Work out the finished part from the listing and answer in its coordinate system (mm). A direction names the side the tool comes from. Coordinates: 2 decimals unless noted, no trailing zeros. Loops run counter-clockwise (first coordinate to the right, second up) from the corner with the lowest first, then second, coordinate; pieces in that order, holes last. Notation, with made-up numbers: M 7.5,-9 L 65.5,-9 A31 cw 65.5,19 Z; hole C -19,44 d9. An arc over 180 degrees is marked long. Write each question's results on one line, items separated by ' | '.
```python
from build123d import *

# Parameters (mm, degrees)
EXTRUDE2_DEPTH = 1.27
EXTRUDE3_DEPTH = 1.27
EXTRUDE4_DEPTH = 1.27


with BuildPart() as part:
    # Sketch2 → Extrude2 (new body)
    with BuildSketch(Plane.XY):
        with BuildLine():
            Line((25.4, 0), (167.299096948, 0))
            Line((167.299096948, 0), (167.299096948, 50.8))
            Line((167.299096948, 50.8), (25.4, 50.8))
            ThreePointArc((25.4, 50.8), (0, 25.4), (25.4, 0))
        make_face()
    extrude(amount=EXTRUDE2_DEPTH)

    # Sketch5 → Extrude3 (add)
    with BuildSketch(Plane.XY.offset(1.27)):
        with BuildLine():
            Line((25.4, 50.8), (37.759096935, 50.8))
            Line((37.759096935, 50.8), (36.934864936, 31.759918178))
            Line((36.934864936, 31.759918178), (25.187364936, 31.759918178))
            ThreePointArc((25.187364936, 31.759918178), (18.674313706, 25.683931539), (24.624718961, 19.055950907))
            Line((24.624718961, 19.055950907), (36.384918961, 19.055950907))
            Line((36.384918961, 19.055950907), (35.56, 0))
            Line((35.56, 0), (25.4, 0))
            ThreePointArc((25.4, 0), (0, 25.4), (25.4, 50.8))
        make_face()
    extrude(amount=EXTRUDE3_DEPTH)

    # Sketch5<4> → Extrude4 (add)
    with BuildSketch(Plane.XY.offset(1.27)):
        with BuildLine():
            Line((153.939033989, 35.56), (166.639033989, 35.56))
            Line((166.639033989, 35.56), (167.299096935, 50.8))
            Line((167.299096935, 50.8), (151.568912005, 50.8))
            ThreePointArc((151.568912005, 50.8), (144.541778303, 47.977914686), (141.418418385, 41.079407862))
            Line((141.418418385, 41.079407862), (141.206176472, 36.176536601))
            ThreePointArc((141.206176472, 36.176536601), (141.660521084, 32.217758839), (143.31923128, 28.594634375))
            Line((143.31923128, 28.594634375), (152.200348571, 15.24))
            Line((152.200348571, 15.24), (139.500348571, 15.24))
            Line((139.500348571, 15.24), (138.840285624, 0))
            Line((138.840285624, 0), (155.369404166, 0))
            ThreePointArc((155.369404166, 0), (162.396457641, 2.822008486), (165.519888176, 9.720370185))
            Line((165.519888176, 9.720370185), (165.683377481, 13.495126865))
            ThreePointArc((165.683377481, 13.495126865), (165.229082159, 17.454048315), (163.570334687, 21.077306532))
            Line((163.570334687, 21.077306532), (153.939033989, 35.56))
        make_face()
        Polygon((53.34, 50.8), (40.64, 50.8), (38.440216103, -0.015869084), (51.140216103, -0.015869084), (51.965822026, 19.055950907), (54.505822026, 19.055950907), (53.680316159, -0.013557756), (66.380816438, -0.002001116), (68.58, 50.8), (55.88, 50.8), (55.055768, 31.759918178), (52.515768, 31.759918178), align=None)
        Polygon((83.479096935, 50.8), (70.779096935, 50.8), (68.58, 0), (81.28, 0), align=None)
        Polygon((111.419096935, 50.8), (86.019096935, 50.8), (83.82, 0), (109.22, 0), (109.846156204, 14.464453409), (97.146156204, 14.464453409), (97.306540074, 18.16938358), (110.006540074, 18.16938358), (110.632696278, 32.633836988), (97.932696278, 32.633836988), (98.093080148, 36.33876716), (110.793080148, 36.33876716), align=None)
        Polygon((139.318340653, 50.8), (113.959096935, 50.8), (111.76, 0), (123.65404294, 0), (124.753591407, 25.4), (138.218792185, 25.4), (138.658714454, 35.562376595), (125.193513676, 35.562376595), (125.413217607, 40.637623405), (138.878418385, 40.637623405), align=None)
    extrude(amount=EXTRUDE4_DEPTH)


solid = part.part
```
1) Find section B-B, the plane z = 0.55. Give the vertices of the cut face in (x, y), and give its area (3 significant figures).
Check result:
outline: M 25.4,0 L 167.3,0 L 167.3,50.8 L 25.4,50.8 A25.4 ccw Z | area: 8,220 mm^2
2) Given pin 1 Ø1.7 at (x, y) = (52.5, 11) entering from +Z; pin 2 Ø1.3 at (x, z) = (78.5, 2) entering from -Y; pin 3 Ø0.6 at (x, z) = (53, 2) entering from -Y, each flat-ended and moving along its own axis, determine where each tip first touches the part or whether it passes through.
Check result:
pin 1: z = 1.27 | pin 2: y = 0 | pin 3: y = 19.06
3) Which of the six approach directions +Z, -Z, +X, -X, +Y, -Y give full straight-line access (tool end or side, diameter ignored) to faces 5 (the face through (162.32, 2.75, 1.9)), 6 (the face through (147.7, 22.01, 1.9)), 7 (the face through (144.62, 48.05, 1.9)), 8 (the face through (122, 31, 2.54)), 9 (the face through (164, 24, 1.27))?
Check result:
face 5: +Z, +X, -Y | face 6: +Z | face 7: +Z, +Y | face 8: +Z, +X, -X, +Y, -Y | face 9: +Z, +X
4) For a pull along X with two mould halves and no side action, classify faces 1 (the face through (158.82, 28.22, 1.9)), 2 (the face through (54, 41, 1.27)), 3 (the face through (15, 26, 2.54)), 4 (the face through (135, 20, 1.27)) as released by +X, released by -X, zero draft, split by the parting line, or undercut.
Check result:
face 1: released by +X | face 2: undercut | face 3: zero draft | face 4: undercut
5) Straight lines are drawn through the part: probe 1 along Y at (x, z) = (102, 2.25); probe 2 along X at (y, z) = (27, 2.2); probe 3 along Y at (x, z) = (142.5, 2.45). For each, find the intervals that lie inside material, in ascending order. Write a range as [from, to].
Check result:
probe 1: [0, 14.46], [18.17, 32.63], [36.34, 50.8] | probe 2: [0.05, 18.87], [39.61, 67.55], [69.75, 82.45], [84.99, 110.39], [112.93, 138.29], [144.38, 159.63] | probe 3: [0, 15.24], [30.02, 45.22]
6) Find section A-A, the plane x = 136.5. Give the vertices of the cut face in (y, z).
Check result:
outline: M 0,0 L 50.8,0 L 50.8,2.54 L 40.64,2.54 L 40.64,1.27 L 35.56,1.27 L 35.56,2.54 L 25.4,2.54 L 25.4,1.27 L 0,1.27 Z
